from build123d import *

# Parameters (mm, degrees)
SKETCH1_R           = 3
BOSS_EXTRUDE1_DEPTH = 12
SKETCH4_W           = 3.217642032
SKETCH4_H           = 5.196152422
CUT_EXTRUDE1_DEPTH  = 10
FILLET1_R           = 0.5


with BuildPart() as part:
    # Sketch1 → Boss-Extrude1 (new body)
    with BuildSketch(Plane(origin=(0, 0, 0), x_dir=(1, 0, 0), z_dir=(0, 1, 0))):
        Circle(SKETCH1_R)
    extrude(amount=BOSS_EXTRUDE1_DEPTH)

    # Sketch4 → Cut-Extrude1 (cut)
    with BuildSketch(Plane(origin=(0, 12, 0), x_dir=(1, 0, 0), z_dir=(0, 1, 0))):
        with Locations((-3.108821016, 0)):
            Rectangle(SKETCH4_W, SKETCH4_H)
    extrude(amount=-CUT_EXTRUDE1_DEPTH, mode=Mode.SUBTRACT)

    # Fillet1
    fillet1_edges = [part.edges().sort_by_distance(p)[0] for p in [
        (1.5, 12, 2.598076211),
        (-1.5, 12, 0),
    ]]
    fillet(fillet1_edges, radius=FILLET1_R)


solid = part.part
Verification items for the finished model (mm, model axes). A direction names the side the tool comes from. Round coordinates to 2 decimals unless told otherwise and drop trailing zeros. Loops run counter-clockwise (first coordinate to the right, second up) from the corner with the lowest first, then second, coordinate; pieces in that order, holes last. Notation, with made-up numbers: (70.5, -32.5) - (109.5, -32.5) arc R33 cw to (109.5, -4.5) - close; hole circle Ø10 at (-13.5, 72.25). An arc over 180 degrees is marked (long way). Use a Markdown table: item, result. Add a question column.
1. Gauge pin test, flat ends, axial feed: pin 1 (3 mm diameter, centred on y = 7, z = 0.5, fed in from +X); pin 2 (1.5 mm diameter, centred on y = 2.5, z = 1.5, fed in from +X); pin 3 (1.5 mm diameter, centred on y = 4, z = -0.5, fed in from -X); pin 4 (1.7 mm diameter, centred on x = -2, z = 0, fed in from +Y). Record the tip position at first contact, or that the pin passes through.
2. Section check A-A, the plane z = 0. Record the boundary of the cut face in (x, y), plus the area to 3 significant figures.
3. Access from +Z, -Z, +X, -X, +Y, -Y to the whole of each face (thin tool, end or side, straight path). Record for faces 1 (the face through (2.86, 5.67, -0.9)), 2 (the face through (-2, 2, 0)).
4. Section check B-B, the plane y = 1. Record the boundary of the cut face in (x, z), plus the area to 3 significant figures.
5. Thickness scan on probe 1 along X at (y, z) = (8.5, 0); probe 2 along Y at (x, z) = (-2, 1.5); probe 3 along Y at (x, z) = (-0.5, 2.5). Record the ranges inside material, lowest first. Write a range as [from, to].
Checks:
| question | item | result |
|---|---|---|
| 1 | pin 1 | stops at x = 3 |
| 1 | pin 2 | stops at x = 2.9 |
| 1 | pin 3 | stops at x = -1.5 |
| 1 | pin 4 | stops at y = 11.98 |
| 2 | outline | (-3, 0) - (3, 0) - (3, 11.5) arc R0.5 ccw to (2.5, 12) - (-1, 12) arc R0.5 ccw to (-1.5, 11.5) - (-1.5, 2) - (-3, 2) - close |
| 2 | area | 56.9 mm^2 |
| 3 | face 1 | +Y, -Y |
| 3 | face 2 | +Z, -Z, -X, +Y |
| 4 | outline | circle Ø6 at (0, 0) |
| 4 | area | 28.3 mm^2 |
| 5 | probe 1 | x = [-1.5, 3] |
| 5 | probe 2 | y = [0, 2] |
| 5 | probe 3 | y = [0, 12] |
